Input: dimensioned drawing with shaded views. Units: mm. Origin: part minimum x, y, z. Coordinates: 2 decimals unless noted, no trailing zeros. Order: outer loops, then holes, each group sorted by start corner. A loop starts at its lowest first (then second) coordinate and runs counter-clockwise, first axis right, second up. Notation, with made-up numbers: M 30,29.25 L 88,29.25 A13 ccw 88,38.25 Z; hole C 28,-34.5 d5. An arc over 180 degrees is marked long. Write item = value, one per line.
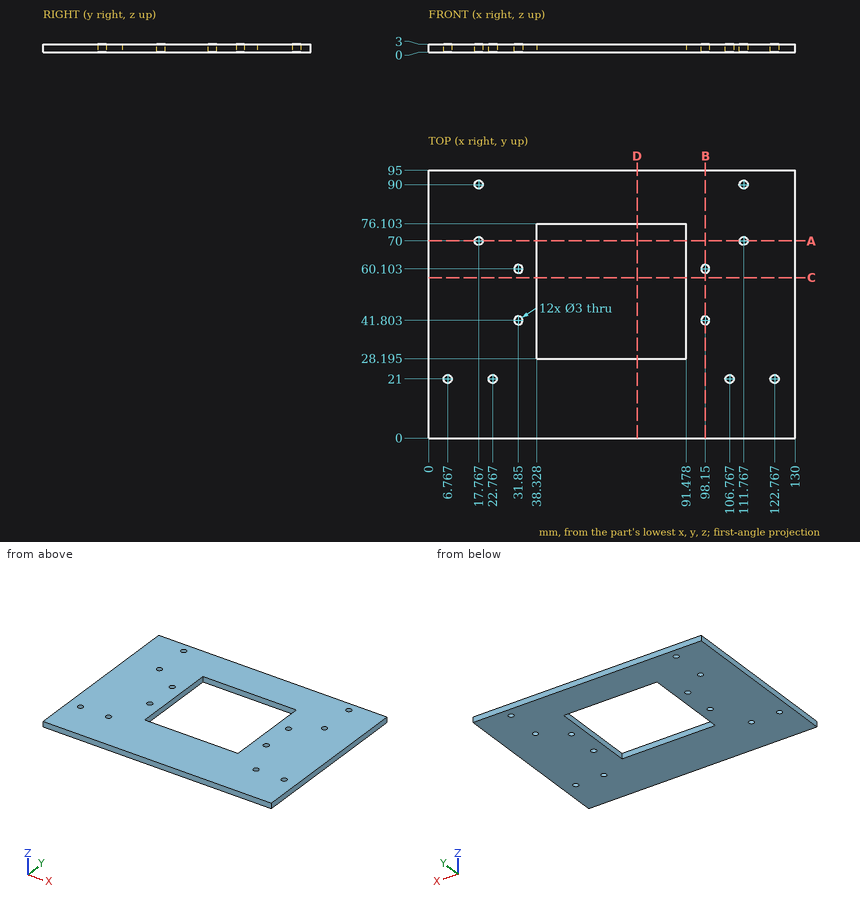
1) Section A-A, the plane y = 70. Return loops of the section in (x, z).
Numbers:
outline = M 0,0 L 16.27,0 L 16.27,3 L 0,3 Z; M 19.27,0 L 38.33,0 L 38.33,3 L 19.27,3 Z; M 91.48,0 L 110.27,0 L 110.27,3 L 91.48,3 Z; M 113.27,0 L 130,0 L 130,3 L 113.27,3 Z
2) Section D-D, the plane x = 74. Return loops of the section in (y, z) (1 decimal).
Numbers:
outline = M 0,0 L 28.2,0 L 28.2,3 L 0,3 Z; M 76.1,0 L 95,0 L 95,3 L 76.1,3 Z
3) Section B-B, the plane x = 98.15. Return loops of the section in (y, z).
Numbers:
outline = M 0,0 L 40.3,0 L 40.3,3 L 0,3 Z; M 43.3,0 L 58.6,0 L 58.6,3 L 43.3,3 Z; M 61.6,0 L 95,0 L 95,3 L 61.6,3 Z
4) Line query: L1, parallel to Y at x = 98.15, z = 2; L2, parallel to X at y = 90, z = 1.4; L3, parallel to Y at x = 112, z = 1.6. Output: solid intervals per line, ascending.
Numbers:
L1 = 0 to 40.3, 43.3 to 58.6, 61.6 to 95
L2 = 0 to 16.27, 19.27 to 110.27, 113.27 to 130
L3 = 0 to 68.52, 71.48 to 88.52, 91.48 to 95
5) Section C-C, the plane y = 57. Return loops of the section in (x, z).
Numbers:
outline = M 0,0 L 38.33,0 L 38.33,3 L 0,3 Z; M 91.48,0 L 130,0 L 130,3 L 91.48,3 Z
